Geometry check sheet. Reference: the model listing, model coordinates, mm. A direction names the side the tool comes from. Coordinates: 2 decimals unless noted, no trailing zeros. Loops run counter-clockwise (first coordinate to the right, second up) from the corner with the lowest first, then second, coordinate; pieces in that order, holes last. Notation, with made-up numbers: (-9.75, -26.75) - (43.25, -26.75) arc R12 cw to (43.25, -14.75) - close; hole circle Ø7 at (24, 62.5). An arc over 180 degrees is marked (long way). One line per item, written item: value.
from build123d import *

# Parameters (mm, degrees)
F0_W           = 80.5555507541
F0_H           = 80
F1_DEPTH       = 175
F2_R           = 32.5
F3_DEPTH       = 300
F4_W           = 25
F4_H           = 300
F5_DEPTH       = 80.001
F6_W           = 300
F6_H           = 25
F7_DEPTH       = 80.5565507541
F8_W           = 80.5555507541
F8_H           = 48.411038518
F9_DEPTH       = 25
F10_R          = 14.0956143059
F11_DEPTH      = 25.001
F13_W          = 80.5555507541
F13_H          = 50
F14_DEPTH      = 10
F14_DEPTH_BACK = 62.5
F15_DEPTH      = 25
F17_DEPTH      = 80.5565507541
F18_R          = 32.5
F19_DEPTH      = 75.001
F20_W          = 3.1050710324
F20_H          = 42.5
F20_W_2        = 40
F21_DEPTH      = 80.5565507541
F22_R          = 12
F23_DEPTH      = 142.501
F24_DEPTH      = 111


with BuildPart() as f1:
    # F0 (on Front) → F1 (new body, symmetric)
    with BuildSketch(Plane.XZ):
        Rectangle(F0_W, F0_H)
    extrude(amount=F1_DEPTH, both=True)

    # F2 (on face) → F3 (cut)
    with BuildSketch(Plane.XZ.offset(175)):
        Circle(F2_R)
    extrude(amount=-F3_DEPTH, mode=Mode.SUBTRACT)

    # F4 (on face) → F5 (cut, through all)
    with BuildSketch(Plane.XY.offset(40)):
        Rectangle(F4_W, F4_H)
    extrude(amount=-F5_DEPTH, mode=Mode.SUBTRACT)

    # F6 (on face) → F7 (cut, through all)
    with BuildSketch(Plane.YZ.offset(40.277775377)):
        Rectangle(F6_W, F6_H)
    extrude(amount=-F7_DEPTH, mode=Mode.SUBTRACT)

    # F8 (on face) → F9 (join)
    with BuildSketch(Plane(origin=(0, 0, -40), x_dir=(1, 0, 0), z_dir=(0, 0, -1))):
        with Locations((0, -199.205519259)):
            Rectangle(F8_W, F8_H)
    extrude(amount=-F9_DEPTH)

    # F10 (on face) → F11 (cut, through all)
    with BuildSketch(Plane.XY.offset(-15)):
        with Locations((0, 199.205519259)):
            Circle(F10_R)
    extrude(amount=-F11_DEPTH, mode=Mode.SUBTRACT)

    # F13 (on offset) → F14 (join, two sides)
    with BuildSketch(Plane.XY.offset(-40)) as f14_sk:
        with Locations((0, 125)):
            Rectangle(F13_W, F13_H)
    extrude(amount=F14_DEPTH)
    extrude(f14_sk.sketch, amount=-F14_DEPTH_BACK)

    # F15 (cut): a face of the model
    f15_faces = [f1.faces().sort_by_distance(p)[0] for p in [
        (0, 175.9398311235, -15),
    ]]
    extrude(f15_faces, amount=-F15_DEPTH, mode=Mode.SUBTRACT)

    # F16 (on face) → F17 (cut, through all)
    with BuildSketch(Plane.YZ.offset(40.277775377)):
        Polygon((100, 79.5669853687), (-178.8060516119, 79.5669853687), (-178.8060516119, -116.9548779726), (100, -116.9548779726), (100, -102.5), (100, -40), (-175, -40), (-175, 40), (100, 40), align=None)
        Polygon((100, 12.5), (100, 40), (-175, 40), (-175, -40), (100, -40), (100, -12.5), (-150, -12.5), (-150, 12.5), align=None)
    extrude(amount=-F17_DEPTH, mode=Mode.SUBTRACT)

    # F18 (on face) → F19 (cut, through all)
    with BuildSketch(Plane(origin=(0, 175, 0), x_dir=(-1, 0, 0), z_dir=(0, 1, 0))):
        Circle(F18_R)
    extrude(amount=-F19_DEPTH, mode=Mode.SUBTRACT)

    # F20 (on face) → F21 (cut, through all)
    with BuildSketch(Plane.YZ.offset(40.277775377)):
        with Locations((98.4474644838, -71.25)):
            Rectangle(F20_W, F20_H)
        with Locations((120, -71.25)):
            Rectangle(F20_W_2, F20_H)
    extrude(amount=-F21_DEPTH, mode=Mode.SUBTRACT)

    # F22 (on face) → F23 (cut, through all)
    with BuildSketch(Plane(origin=(0, 0, -102.5), x_dir=(1, 0, 0), z_dir=(0, 0, -1))):
        with Locations((0, -125)):
            Circle(F22_R)
    extrude(amount=-F23_DEPTH, mode=Mode.SUBTRACT)

    # F17_face (on face) + F21_face (on face) → F24 (join)
    with BuildSketch(Plane(origin=(-28.870034174, 100, 28.6839226626), x_dir=(1, 0, 0), z_dir=(0, -1, 0))):
        with BuildLine():
            ThreePointArc((-1.129965826, -16.1839226626), (5.8890637854, -5.7029522741), (16.370034174, 1.3160773374))
            Line((16.370034174, 1.3160773374), (16.370034174, 11.3160773374))
            Line((16.370034174, 11.3160773374), (-11.4077412031, 11.3160773374))
            Line((-11.4077412031, 11.3160773374), (-11.4077412031, -16.1839226626))
            Line((-11.4077412031, -16.1839226626), (-1.129965826, -16.1839226626))
        make_face()
        with BuildLine():
            Line((69.147809551, -16.1839226626), (69.147809551, 11.3160773374))
            Line((69.147809551, 11.3160773374), (41.370034174, 11.3160773374))
            Line((41.370034174, 11.3160773374), (41.370034174, 1.3160773374))
            ThreePointArc((41.370034174, 1.3160773374), (51.8510045625, -5.7029522741), (58.870034174, -16.1839226626))
            Line((58.870034174, -16.1839226626), (69.147809551, -16.1839226626))
        make_face()
    with BuildSketch(Plane(origin=(0, 100, -35.4746848598), x_dir=(1, 0, 0), z_dir=(0, -1, 0))):
        with BuildLine():
            Line((-40.277775377, 22.9746848598), (-40.277775377, -14.5253151402))
            Line((-40.277775377, -14.5253151402), (40.277775377, -14.5253151402))
            Line((40.277775377, -14.5253151402), (40.277775377, 22.9746848598))
            Line((40.277775377, 22.9746848598), (30, 22.9746848598))
            ThreePointArc((30, 22.9746848598), (0, 2.9746848598), (-30, 22.9746848598))
            Line((-30, 22.9746848598), (-40.277775377, 22.9746848598))
        make_face()
    extrude(amount=F24_DEPTH)


solid = f1.part
(1) Material ranges on probe 1 along Y at (x, z) = (0, -41); probe 2 along X at (y, z) = (125, -96.75); probe 3 along X at (y, z) = (151, 0), recorded low to high. Write a range as from..to.
Reply:
probe 1: -11..113, 137..150
probe 2: -40.28..-12, 12..40.28
probe 3: -40.28..-32.5, 32.5..40.28
(2) Cross-section at A-A on y = 78.5. Record the cut outline in (x, z).
Reply:
outline: (-40.28, -50) - (40.28, -50) - (40.28, -12.5) - (30, -12.5) arc R32.5 cw to (-30, -12.5) - (-40.28, -12.5) - close; (-40.28, 12.5) - (-30, 12.5) arc R32.5 cw to (-12.5, 30) - (-12.5, 40) - (-40.28, 40) - close; (12.5, 30) arc R32.5 cw to (30, 12.5) - (40.28, 12.5) - (40.28, 40) - (12.5, 40) - close
(3) Release check for a two-part mould opening along Y. For faces 6 (the face through (-1, 162, -40)), 7 (the face through (-11.99, 124.47, -40.24)), 8 (the face through (36, 150, 0)) record: pulls with the +Y half, pulls with the -Y half, needs draft (parallel to the pull), parting line crosses it, or undercut.
Reply:
face 6: needs draft
face 7: undercut
face 8: pulls with the -Y half
(4) Cross-section at C-C on x = 0. Record the cut outline in (y, z).
Reply:
outline: (-11, -50) - (113, -50) - (113, -32.5) - (-11, -32.5) - close; (100, -102.5) - (113, -102.5) - (113, -92.5) - (100, -92.5) - close; (137, -102.5) - (150, -102.5) - (150, -40) - (175, -40) - (175, -32.5) - (137, -32.5) - (137, -50) - (140, -50) - (140, -92.5) - (137, -92.5) - close; (150, 32.5) - (175, 32.5) - (175, 40) - (150, 40) - close
(5) Access from +Z, -Z, +X, -X, +Y, -Y to the whole of each face (thin tool, end or side, straight path). Record for faces 1 (the face through (-18.5, 175, 27.2)), 2 (the face through (0, 150, 36)), 3 (the face through (-1, 150, -71)), 4 (the face through (-36, 150, 0)), 5 (the face through (1, 100, -98)).
Reply:
face 1: +Z, -Z, +X, -X, +Y
face 2: +Z, -Y
face 3: -Z, +X, -X, +Y
face 4: +X, -X, -Y
face 5: -Z, +X, -X, -Y
(6) Cross-section at D-D on x = -16. Record the cut outline in (y, z), and give its area (3 significant figures).
Reply:
outline: (-11, -50) - (140, -50) - (140, -92.5) - (100, -92.5) - (100, -102.5) - (150, -102.5) - (150, -40) - (175, -40) - (175, -28.29) - (-11, -28.29) - close; (-11, 28.29) - (175, 28.29) - (175, 40) - (-11, 40) - close
area: 6,890 mm2
(7) Go/stop test with flat-tipped pins: pin 1 Ø3 at (x, z) = (4, 33) entering from -Y; pin 2 Ø7.5 at (x, y) = (7, 166.5) entering from -Z; pin 3 Ø3 at (x, z) = (-9.5, -97) entering from -Y. Record where each tip stops, or that it passes through.
Reply:
pin 1: y = 150
pin 2: z = -40
pin 3: y = 100
(8) Cross-section at B-B on z = 0. Record the cut outline in (x, y), and give its area (3 significant figures).
Reply:
outline: (-40.28, 150) - (-32.5, 150) - (-32.5, 175) - (-40.28, 175) - close; (32.5, 150) - (40.28, 150) - (40.28, 175) - (32.5, 175) - close
area: 389 mm2
